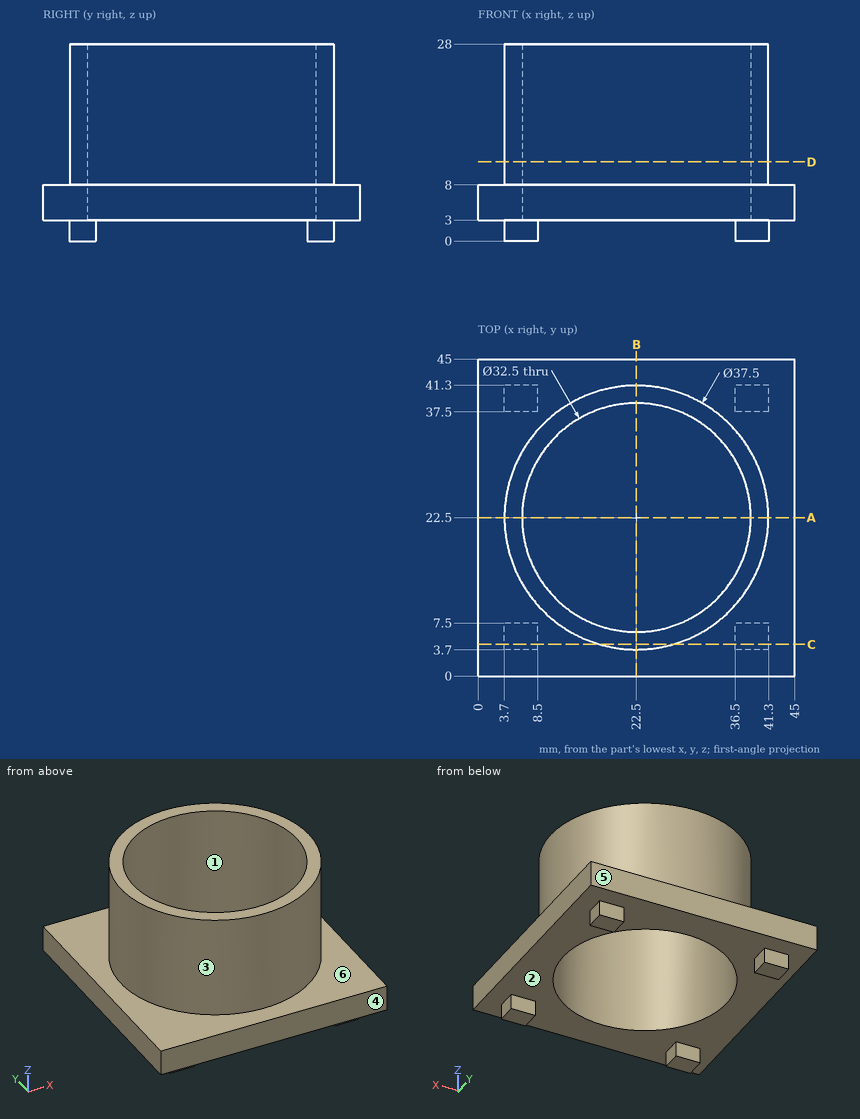
Answer from the drawing. Dimensions are ordinates in mm from the lowest x, y and z of the part. A direction names the side the tool comes from. Give positions to 0.01 mm unless a question says otherwise; leave off trailing zeros. Loops run counter-clockwise (first coordinate to the right, second up) from the corner with the lowest first, then second, coordinate; pieces in that order, holes last. Notation, with made-up numbers: (77.5, -32.75) - (113.5, -32.75) arc R27 ccw to (113.5, 3.25) - close; hole circle Ø7 at (49.25, 36.25). An arc over 180 degrees is marked (long way). Write each question's results on one line, items separated by ' | '.
1. Consider probe 1 along Y at (x, z) = (22.5, 21); probe 2 along X at (y, z) = (35, 10.5); probe 3 along Z at (x, y) = (42, 6.5). Determine where each line is inside the solid, lowest interval first. Write a range as from..to.
Resolved:
probe 1: y = 3.75..6.25, 38.75..41.25 | probe 2: x = 8.52..12.12, 32.88..36.48 | probe 3: z = 3..8
2. Flat-ended cylindrical pins translate along their axes: P1, Ø1.5, axis at y = 40, z = 1, coming from the +X side; P2, Ø2.5, axis at y = 39, z = 1, coming from the -X side; P3, Ø3.5, axis at x = 39.5, z = 1, coming from the +Y side. Find the tip coordinate at first contact, or state that the pin passes through.
Resolved:
P1: stops at x = 41.3 | P2: stops at x = 3.7 | P3: stops at y = 41.3
3. For a pull along Y with two mould halves and no side action, classify the marked faces 1, 2, 3 and 4 as +Y half, -Y half, draft (parallel to the pull), parting line (faces both ways), or undercut.
Resolved:
face 1: undercut | face 2: undercut | face 3: parting line | face 4: -Y half
4. Find section C-C, the plane y = 4.5. Write down the section's boundary in (x, z), then the cut area to 3 significant figures.
Resolved:
outline: (0, 3) - (3.7, 3) - (3.7, 0) - (8.5, 0) - (8.5, 3) - (36.5, 3) - (36.5, 0) - (41.3, 0) - (41.3, 3) - (45, 3) - (45, 8) - (27.75, 8) - (27.75, 28) - (17.25, 28) - (17.25, 8) - (0, 8) - close | area: 464 mm^2
5. Find section A-A, the plane y = 22.5. Write down the section's boundary in (x, z), then the cut area to 4 significant figures.
Resolved:
outline: (0, 3) - (6.25, 3) - (6.25, 28) - (3.75, 28) - (3.75, 8) - (0, 8) - close; (38.75, 3) - (45, 3) - (45, 8) - (41.25, 8) - (41.25, 28) - (38.75, 28) - close | area: 162.5 mm^2
6. Which of the six approach directions +Z, -Z, +X, -X, +Y, -Y give full straight-line access (tool end or side, diameter ignored) to the marked faces 5 and 6?
Resolved:
face 5: +Z, -Z, +X, -X, +Y | face 6: +Z
7. Find section D-D, the plane z = 11.25. Write down the section's boundary in (x, y), then the cut area to 3 significant figures.
Resolved:
outline: circle Ø37.5 at (22.5, 22.5); hole circle Ø32.5 at (22.5, 22.5) | area: 275 mm^2
